from build123d import *

# Parameters (mm, degrees)
SKETCH1_R           = 2.555
BOSS_EXTRUDE1_DEPTH = 5
FILLET1_R           = 4
CUT_EXTRUDE1_START  = -2
CUT_EXTRUDE1_DEPTH  = 2
FILLET3_R           = 0.5


with BuildPart() as part:
    # Sketch1 → Boss-Extrude1 (new body)
    with BuildSketch(Plane(origin=(0, 0, 0), x_dir=(1, 0, 0), z_dir=(0, 1, 0))):
        with BuildLine():
            Line((-5, 0), (-5, 23.957730656))
            ThreePointArc((-5, 23.957730656), (9.365764476, 22.610955619), (20.476207715, 13.405139903))
            Line((20.476207715, 13.405139903), (3.535533906, -3.535533906))
            ThreePointArc((3.535533906, -3.535533906), (-1.913417162, -4.619397663), (-5, 0))
        make_face()
        with Locations(Location((0, 0, 0), (0, 0, 270))):
            Circle(SKETCH1_R, mode=Mode.SUBTRACT)
        with Locations(Location((7.071067812, 7.071067812, 0), (0, 0, 270))):
            Circle(SKETCH1_R, mode=Mode.SUBTRACT)
        with BuildLine():
            ThreePointArc((0, 21.973922003), (-1.15, 20.823922003), (0, 19.673922003))
            ThreePointArc((0, 19.673922003), (7.528884, 18.176333863), (13.911563661, 13.911563661))
            ThreePointArc((13.911563661, 13.911563661), (15.537909258, 13.911563661), (15.537909258, 15.537909258))
            ThreePointArc((15.537909258, 15.537909258), (8.409055895, 20.301256788), (0, 21.973922003))
        make_face(mode=Mode.SUBTRACT)
    extrude(amount=BOSS_EXTRUDE1_DEPTH)

    # Fillet1
    fillet1_edges = [part.edges().sort_by_distance(p)[0] for p in [
        (-5, 2.5, -23.957730656),
        (20.476207715, 2.5, -13.405139903),
    ]]
    fillet(fillet1_edges, radius=FILLET1_R)

    # Sketch2 → Cut-Extrude1 (cut)
    # profile 1 of 3: a face of its own
    with BuildSketch(Plane(origin=(0, 5, 0), x_dir=(1, 0, 0), z_dir=(0, 1, 0)).offset(CUT_EXTRUDE1_START)):
        with BuildLine():
            ThreePointArc((17.995504206, 10.924436395), (18.929126851, 12.393826533), (19.150132948, 14.120648738))
            ThreePointArc((19.150132948, 14.120648738), (16.926987938, 10.570555283), (12.842220443, 11.498031317))
            ThreePointArc((12.842220443, 11.498031317), (14.122014888, 9.884130998), (15.200167421, 8.129099609))
            Line((15.200167421, 8.129099609), (17.995504206, 10.924436395))
        make_face()
    # profile 2 of 3: a face of its own
    with BuildSketch(Plane(origin=(0, 5, 0), x_dir=(1, 0, 0), z_dir=(0, 1, 0)).offset(CUT_EXTRUDE1_START)):
        with BuildLine():
            ThreePointArc((19.150132948, 14.120648738), (18.82866037, 15.363083326), (18.130276234, 16.439767087))
            ThreePointArc((18.130276234, 16.439767087), (9.365764476, 22.610955619), (-1.195370482, 24.444712058))
            ThreePointArc((-1.195370482, 24.444712058), (-2.450533029, 24.177213828), (-3.556382391, 23.525995345))
            ThreePointArc((-3.556382391, 23.525995345), (-4.494676634, 19.443699277), (-0.950485246, 17.211157075))
            ThreePointArc((-0.950485246, 17.211157075), (6.59646064, 15.925264742), (12.842220443, 11.498031317))
            ThreePointArc((12.842220443, 11.498031317), (16.926987938, 10.570555283), (19.150132948, 14.120648738))
        make_face()
        with BuildLine():
            ThreePointArc((0, 19.673922003), (-1.15, 20.823922003), (0, 21.973922003))
            ThreePointArc((0, 21.973922003), (8.409055895, 20.301256788), (15.537909258, 15.537909258))
            ThreePointArc((15.537909258, 15.537909258), (15.537909258, 13.911563661), (13.911563661, 13.911563661))
            ThreePointArc((13.911563661, 13.911563661), (7.528884, 18.176333863), (0, 19.673922003))
        make_face(mode=Mode.SUBTRACT)
    # profile 3 of 3: a face of its own
    with BuildSketch(Plane(origin=(0, 5, 0), x_dir=(1, 0, 0), z_dir=(0, 1, 0)).offset(CUT_EXTRUDE1_START)):
        with BuildLine():
            ThreePointArc((-0.950485246, 17.211157075), (-4.494676634, 19.443699277), (-3.556382391, 23.525995345))
            ThreePointArc((-3.556382391, 23.525995345), (-4.621155172, 22.148672745), (-5, 20.44948611))
            Line((-5, 20.44948611), (-5, 16.496282917))
            ThreePointArc((-5, 16.496282917), (-2.996636437, 16.974908546), (-0.950485246, 17.211157075))
        make_face()
    extrude(amount=CUT_EXTRUDE1_DEPTH, mode=Mode.SUBTRACT)

    # Fillet3
    fillet3_edges = [part.edges().sort_by_distance(p)[0] for p in [
        (-1.913417162, 5, 4.619397663),
        (-5, 5, -8.248141459),
        (19.165883391, 3, -13.655149118),
        (16.597835814, 3, -9.526768002),
        (6.59646064, 3, -15.925264742),
        (15.200167421, 4, -8.129099609),
        (-5, 3, -18.472884514),
        (-5, 4, -16.496282917),
        (-3.896677573, 3, -23.207974653),
        (9.365764476, 3, -22.610955619),
        (6.59646064, 5, -15.925264742),
        (9.367850663, 5, -2.296782852),
    ]]
    fillet(fillet3_edges, radius=FILLET3_R)


solid = part.part
Can you work these out from the model? Positions are in its coordinate system, mm. A direction names the side the tool comes from. Give positions to 0.01 mm unless a question says otherwise; leave off trailing zeros. One line per item, written item: value.
1) Imagine slicing it at A-A on y = 1.85. Count the separate pieces of the cut face and the enclosed holes in it, and give its area (3 significant figures).
Geometry check:
separate pieces: 1
enclosed holes: 3
area: 420 mm²
2) I'm going to push a flat-ended pin straight in: pin 1 (1.5 mm diameter, centred on x = 10, z = -0.5, fed in from +Y). Where does the tip first touch, or does it pass through?
Geometry check:
pin 1: passes through
3) On a 3-axis mill with a long thin cutter (end or side, diameter ignored), from which of +Z, -Z, +X, -X, +Y, -Y can I reach the whole of each face in a straight line? I mean faces 4 (the face through (-1.15, 1.48, -20.85)), 5 (the face through (-3.926, 1.268, -23.177)). Say none if no direction works.
Geometry check:
face 4: +Y, -Y
face 5: -Z, -X, +Y, -Y
4) Please list where these lines run through material, in increasing order: line 1 (Z direction, x = 8.25, y = 2.85); line 2 (Z direction, x = 7.25, y = 2.75); line 3 (Z direction, x = 12.5, y = 2.8).
Geometry check:
line 1: z = -22.89 to -20.37, -17.86 to -9.34, -4.8 to -1.18
line 2: z = -23.31 to -20.74, -18.29 to -9.62, -4.52 to -0.18
line 3: z = -20.92 to -18.07, -15.19 to -5.43
5) Thinking about a two-plate mould opening in X: for faces 1 (the face through (-1.84, 2.22, 4.65)), 2 (the face through (7.429, 1.479, -18.217)), 3 (the face through (3, 5, -9)), which applies, +X half, -X half, draft (parallel to the pull), parting line (faces both ways), or undercut?
Geometry check:
face 1: parting line
face 2: undercut
face 3: draft
